Autodesk Fusion 360 part; units mm, degrees
sketch "Sketch4" plane through (0, 0, 0) normal (0, 0, 1) x (-1, 0, 0)
  circle A0 centre (-15.6, 0) radius 2.5
  line L0 (3.7, 0) -> (-18.1, 0) construction
  circle A1 centre (0, 0) radius 3.7
  line L1 (0, 0) -> (0, -3.7) construction
  line L2 (0, 0) -> (0, 3.7) construction
  line L3 (-15.6, 0) -> (-15.6, -2.5) construction
  line L4 (-15.6, 0) -> (-15.6, 2.5) construction
  line L5 (-15.6, -2.5) -> (0, -3.7)
  line L6 (-15.6, 2.5) -> (0, 3.7)
  circle A2 centre (0, 0) radius 1.35
  circle A3 centre (0, 0) radius 2.3
  circle A4 centre (-15.6, 0) radius 0.2875
  circle A5 centre (-13.55, 0) radius 0.2875
  circle A6 centre (-11.5, 0) radius 0.2875
  circle A7 centre (-9.45, 0) radius 0.2875
  circle A8 centre (-7.4, 0) radius 0.2875
  circle A9 centre (-5.35, 0) radius 0.2875
  point P0 (-15.6, 0)
  point P1 (-4.9, 0)
  dimension "d12" = 5
  dimension "d13" = 21.8
  dimension "d14" = 3.7
  dimension "d15" = 2.5
  dimension "d16" = 7.4
  dimension "d17" = 2.7
  dimension "d18" = 4.6
  dimension "d24" = 13.2
  dimension "d28" = 0.575
  dimension "d31" = -2.05
  dimension "d32" = 0
extrude "Extrude3" add sketch "Sketch4" along normal blind 5.2 contours A1 L5 L6 | A1 L6 | A1 L5
extrude "Extrude4" add sketch "Sketch4" along normal blind 2.5 from surface at 1.8 contours A0 | A0 A1 L5 L6 | A4 | A5 | A6 | A7 | A8 | A9
extrude "Extrude5" add sketch "Sketch4" along normal blind 1.15 from surface at 2.75 contours A3
extrude "Extrude6" cut sketch "Sketch4" along normal through all contours A4 | A5 | A6 | A7 | A8 | A9
sketch "Sketch5" plane through (0, 0, 4.3) normal (0, 0, 1) x (-1, 0, 0)
  circle A0 centre (-9.45, 0) radius 0.2875
  circle A1 centre (-15.6, 0) radius 0.2875
  circle A2 centre (-7.4, 0) radius 0.2875
  circle A3 centre (-11.5, 0) radius 0.2875
  circle A4 centre (-13.55, 0) radius 0.2875
  circle A5 centre (-5.35, 0) radius 0.2875
  line L0 (-15.6, -2.5) -> (-0.5659, -3.6565)
  arc A6 (-0.5659, 3.6565) -> (-0.5659, -3.6565) centre (0, 0) ccw
  line L1 (-0.5659, 3.6565) -> (-15.6, 2.5)
  arc A7 (-15.6, 2.5) -> (-15.6, -2.5) centre (-15.6, 0) ccw
  line L2 (3.7, 0) -> (-18.1, 0)
  line L3 (-4.9, 0) -> (-4.9, -3.3231) construction
  line L4 (-4.9, 0) -> (-4.9, 3.3231) construction
  line L5 (-4.9, -2.3231) -> (2.8798, -2.3231)
  line L6 (-4.9, -0.5) -> (3.6661, -0.5)
  line L7 (-4.9, 0.5) -> (3.6661, 0.5)
  line L8 (-4.9, 2.3231) -> (2.8798, 2.3231)
  line L9 (-4.9, -3.3231) -> (-4.9, -2.3231)
  line L10 (-4.9, -0.5) -> (-4.9, 0.5)
  line L11 (-4.9, 2.3231) -> (-4.9, 3.3231)
  point P0 (-4.9, 0)
  dimension "d34" = 1
  dimension "d35" = 0.5
  dimension "d36" = 0.5
  dimension "d37" = 1
extrude "Extrude7" add sketch "Sketch5" along normal up to surface (0.9 mm away) contours A6 L2 L7 L10 | A6 L2 L6 L10 | A6 L1 L8 L11 | L0 A6 L5 L9
ref_plane "WorkPlane1" through (4.283, -3.7, 4.75) normal (0, -1, 0) x (1, 0, 0)
sketch "Sketch7" plane through (0, -3.7, 0) normal (0, -1, 0) x (-1, 0, 0)
  line L0 (-4.9, -5.2) -> (-3.6661, -5.2)
  line L1 (-3.6661, -5.2) -> (-3.6661, -4.3)
  line L2 (-3.6661, -4.3) -> (-4.9, -4.3)
  line L3 (-4.9, -4.3) -> (-4.9, -5.2)
  line L4 (-3.6661, -5.2) -> (-4.9, -4.3)
extrude "Extrude8" cut sketch "Sketch7" against normal through all contours L0 L3 L4
equation "d14 = d16 / 2"
equation "d15 = d12 / 2"
equation "d36 = d35"
Part model, mm, in its own coordinate system. A direction names the side the tool comes from. Give positions to 0.01 mm unless a question says otherwise; leave off trailing zeros. Write each loop counter-clockwise with the first axis right and the second up, starting at its lowest first coordinate (ties: lowest second). Pieces come first, ordered by that corner, then holes. Notation, with made-up numbers: (28, 16.25) -> (55, 16.25) arc R37 cw to (55, 55.25) -> close; hole circle Ø10 at (-11.5, -26.5). An arc over 180 degrees is marked (long way). Put each result on its own line as item: value. Start each with the question number.
Item 1: Cut at B-B (x = 13.55). List the corners of the cut face in (y, z).
Item 2: Cut at A-A (z = 3.25). State how many separate pieces and enclosed holes the cut face has, then the cut area to 3 significant figures.
Item 3: Wall check: L1, parallel to Y at x = 0, z = 3.15; L2, parallel to Y at x = 5.35, z = 2.6; L3, parallel to Z at x = 9.5, y = -2.5. Give the ranges that are in metal, low to high. Write a range as [from, to].
Item 4: Pull direction Y, two halves, no side cores. Call faces 4 (the face through (3.7, -2.323, 4.6)), 5 (the face through (2, 2, 5.2)), 6 (the face through (-3.53, 1.11, 1.99)): pulls with the +Y half, pulls with the -Y half, needs draft (parallel to the pull), parting line crosses it, or undercut.
Item 5: Cut at D-D (z = 4.75). List the corners of the cut face in (x, y), then the cut area to 3 significant figures.
Item 6: Pin check, flat tips, straight feed: pin 1 Ø2 at (x, z) = (1.5, 3.5) entering from -Y; pin 2 Ø4 at (x, y) = (0, 0) entering from +Z; pin 3 Ø1.5 at (x, y) = (15, 2.5) entering from -Z. Stop position of each tip, or through.
Item 7: Which spindle directions (+Z, -Z, +X, -X, +Y, -Y) get a long thin tool onto all of the face, cutting with end or side? Do faces 1 (the face through (1.825, -1.4, 4.541)), 2 (the face through (0, 2, 2.75)), 3 (the face through (4.2, -0.5, 4.6)). Say none if no direction does.
Answer list:
1. outline: (-2.66, 1.8) -> (-0.29, 1.8) -> (-0.29, 4.3) -> (-2.66, 4.3) -> close; (0.29, 1.8) -> (2.66, 1.8) -> (2.66, 4.3) -> (0.29, 4.3) -> close
2. separate pieces: 1
2. enclosed holes: 7
2. area: 121 mm2
3. L1: y = [-3.7, -1.35], [1.35, 3.7]
3. L2: y = [-3.29, -0.29], [0.29, 3.29]
3. L3: z = [1.8, 4.3]
4. face 4: undercut
4. face 5: needs draft
4. face 6: parting line crosses it
5. outline: (0.57, -3.66) -> (4.28, -3.37) -> (4.28, -2.32) -> (2.88, -2.32) arc R3.7 ccw to (3.67, -0.5) -> (4.28, -0.5) -> (4.28, 0.5) -> (3.67, 0.5) arc R3.7 ccw to (2.88, 2.32) -> (4.28, 2.32) -> (4.28, 3.37) -> (0.57, 3.66) arc R3.7 ccw (long way) to start; hole circle Ø4.6 at (0, 0)
5. area: 31.9 mm2
6. pin 1: stops at y = -3.67
6. pin 2: stops at z = 3.9
6. pin 3: stops at z = 1.8
7. face 1: +Z
7. face 2: -Z
7. face 3: +Z, +X
